Could you check a few things on this model? Use its own coordinates, in mm. Face numbers are marked on the shaded views. A direction names the side the tool comes from. Give positions to 0.01 mm unless a question says otherwise; leave off trailing zeros. Loops run counter-clockwise (first coordinate to the right, second up) from the corner with the lowest first, then second, coordinate; pieces in that order, holes last.
1. Imagine slicing it at D-D (x = 5). List the corners of the cut face in (y, z) for me.
2. Imagine slicing it at C-C (z = -21). List the corners of the cut face in (x, y) for me.
3. Imagine slicing it at B-B (y = -13). List the corners of the cut face in (x, z) for me.
4. For the marked faces 1, 2, 3 and 4, which set-ups out of +Z, -Z, +X, -X, +Y, -Y let a thin tool reach every point of the face, with its end or its side?
5. Thinking about a two-plate mould opening in Z: for the marked faces 5, 6 and 7, which applies, +Z half, -Z half, draft (parallel to the pull), parting line (faces both ways), or undercut?
6. I need wall thicknesses on line 1 along Y through (x, z) = (13.2, -21); line 2 along Z through (x, y) = (2.25, -5); line 3 along Z through (x, y) = (12.75, 1). Which ranges of each line are inside material? Lowest first, please.
7. Imagine slicing it at A-A (z = -4). List the corners of the cut face in (x, y) for me.
8. For P1, Ø1.2, axis at x = 0, y = 0, coming from the -Z side; P2, Ø3, axis at x = 11.5, z = -7.5, coming from the -Y side; P3, Ø1, axis at x = 9, z = -10, coming from the -Y side; P4, Ø5, axis at y = -13, z = 2, coming from the -X side, each with a flat end and sliding along its axis, tell me the tip position at first contact or that it passes through.
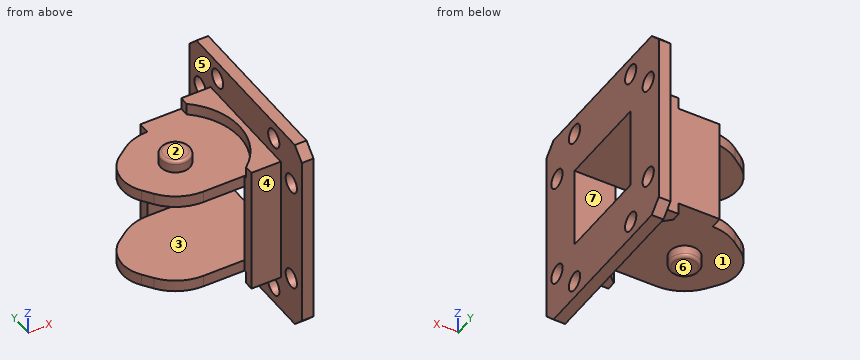
Autodesk Inventor part; units mm, degrees
ref_plane "Work Plane1" through (11, 0, 4) normal (1, 0, 0) x (0, 1, 0)
ref_plane "Work Plane2" through (0, 0, -7) normal (0, 0, -1) x (-1, 0, 0)
ref_plane "YZ Plane" through (0, 0, 0) normal (1, 0, 0) x (0, 1, 0)
sketch "Sketch1" plane through (0, 0, 0) normal (0, 0, 1) x (1, 0, 0)
  circle A0 centre (0, 0) radius 2.5
  circle A1 centre (20, 0) radius 2.5
  line L0 (7, 10) -> (20, 10)
  line L1 (7, -10) -> (20, -10)
  arc A2 (20, -10) -> (20, 10) centre (20, 0) ccw
  line L2 (7, 10) -> (7, 8)
  line L3 (7, -10) -> (7, -8)
  line L4 (7, 8) -> (0, 8)
  line L5 (7, -8) -> (0, -8)
  arc A3 (0, 8) -> (0, -8) centre (0, 0) ccw
  dimension "d0" = 5
  dimension "d1" = 20
  dimension "d2" = 10
  dimension "d3" = 2
  dimension "d4" = 13
extrude "Extrusion1" add sketch "Sketch1" along normal blind 4
sketch "Sketch2" plane through (0, 0, 4) normal (0, 0, 1) x (1, 0, 0)
  circle A0 centre (0, 0) radius 2.5
  line L0 (7, 8) -> (0, 8)
  arc A1 (0, 8) -> (0, -8) centre (0, 0) ccw
  line L1 (0, -8) -> (7, -8)
  line L2 (7, -10) -> (20, -10)
  line L3 (7, 8) -> (7, -8)
  line L4 (7, -8) -> (0, -8)
  line L5 (7, 8) -> (0, 8)
  arc A2 (0, 8) -> (0, -8) centre (0, 0) ccw
extrude "Extrusion2" cut sketch "Sketch2" against normal blind 2
sketch "Sketch3" plane through (0, 0, 0) normal (0, 0, -1) x (-1, 0, 0)
  circle A0 centre (-20, 0) radius 2.5
  circle A1 centre (0, 0) radius 2.5
  line L0 (-7, 10) -> (-20, 10)
  arc A2 (-20, 10) -> (-20, -10) centre (-20, 0) ccw
  line L1 (-20, -10) -> (-7, -10)
  line L2 (-7, 8) -> (-7, 10)
  line L3 (-19, 10) -> (-19, 8)
  line L4 (-19, 8) -> (-11, 8)
  line L5 (-11, 8) -> (-11, -8)
  line L6 (-11, -8) -> (-19, -8)
  line L7 (-19, -8) -> (-19, -10)
  point P0 (-7, -8)
  dimension "d9" = 1
  dimension "d10" = 11
extrude "Extrusion3" cut sketch "Sketch3" against normal blind 2 contours L3 L4 L5 L6 L7 L1 A2 L0
sketch "Sketch4" plane through (0, 0, 4) normal (0, 0, 1) x (1, 0, 0)
  line L0 (7, 10) -> (7, -10)
  circle A0 centre (0, 0) radius 2.5
  arc A1 (7, -8.485281) -> (7, 8.485281) centre (0, 0) ccw
  dimension "d15" = 11
extrude "Extrusion4" cut sketch "Sketch4" against normal blind 2 contours A1 L0
sketch "Sketch5" plane through (0, 0, 0) normal (0, 0, -1) x (-1, 0, 0)
  line L0 (0, 8) -> (-7, 8)
  line L1 (-7, 10) -> (0, 10)
  line L2 (0, 10) -> (0, 8)
  line L3 (0, 8) -> (-7, 8)
  line L4 (-7, 8) -> (-7, 10)
  arc A0 (0, -8) -> (0, 8) centre (0, 0) ccw
extrude "Extrusion5" add sketch "Sketch5" against normal blind 2
sketch "Sketch6" plane through (0, 0, 0) normal (0, 0, -1) x (-1, 0, 0)
  line L0 (0, 10) -> (-19, 10)
  line L1 (-19, 8) -> (-20, 8)
  line L2 (-20, 8) -> (-20, 10)
  line L3 (-20, 10) -> (-19, 10)
  line L4 (-19, 10) -> (-19, 8)
  circle A0 centre (-20, 0) radius 2.5
extrude "Extrusion6" add sketch "Sketch6" against normal blind 2 contours L1 L2 L3 L4
sketch "Sketch7" plane through (0, 0, 0) normal (0, 0, -1) x (-1, 0, 0)
  line L0 (-19, -8) -> (-19, -10)
  line L1 (-11, -8) -> (-19, -8)
  line L2 (-17.400642, -8) -> (-19, -9.162001)
  line L3 (-17.400642, -8) -> (-26.805206, 4.944272) construction
  line L4 (-26.805206, 4.944272) -> (-28.404564, 3.782271) construction
  line L5 (-28.404564, 3.782271) -> (-19, -9.162001) construction
  circle A0 centre (-20, 0) radius 2.5
  line L6 (-17.400642, -8) -> (-19, -8)
  line L7 (-19, -8) -> (-19, -9.162001)
  dimension "d21" = 16
  dimension "d22" = 8
  dimension "d23" = 36
extrude "Extrusion7" cut sketch "Sketch7" against normal blind 2 contours L1 L2 L0
sketch "Sketch9" plane through (0, 0, 2) normal (0, 0, 1) x (1, 0, 0)
  circle A0 centre (0, 0) radius 2.5
  arc A1 (11, 0) -> (7, 8.485281) centre (0, 0) ccw
  circle A2 centre (0, 0) radius 2.5
extrude "Extrusion8" add sketch "Sketch9" along normal mid plane 4
fillet "Fillet1" radius 0.5 1 edges at (-2.5, 0, 4)
sketch "Sketch10" plane through (0, 0, 0) normal (0, 0, -1) x (-1, 0, 0)
  arc A0 (0, -8) -> (0, 8) centre (0, 0) ccw
  line L0 (0, 10) -> (-20, 10)
  line L1 (4.702282, 6.472136) -> (11.174418, 1.769854)
  line L2 (11.174418, 1.769854) -> (6.472136, -4.702282)
  dimension "d30" = 144
extrude "Extrusion9" add sketch "Sketch10" against normal blind 2
fillet "Fillet2" radius 6 1 edges at (-11.1744, 1.7699, 1)
ref_plane "Work Plane1" through (11, 0, 4) normal (1, 0, 0) x (0, 1, 0)
split "Split1" plane through (11, 0, 4) removes the side toward (1, 0, 0)
sketch "Sketch11" plane through (11, -10, 0) normal (1, 0, 0) x (0, 0, -1)
  line L0 (0, 20) -> (0, 0)
  line L1 (-4, 20) -> (0, 20)
  line L2 (-4, 10) -> (-4, 20)
  line L3 (-4, 0) -> (-4, 10)
  line L4 (0, 0) -> (-4, 0)
  point P0 (0, 10)
extrude "Extrusion10" add sketch "Sketch11" along normal blind 1
ref_plane "Work Plane2" through (0, 0, -7) normal (0, 0, -1) x (-1, 0, 0)
mirror "Mirror1" about plane through (0, 0, -7) normal (0, 0, -1)
sketch "Sketch12" plane through (0, 0, 0) normal (0, 0, -1) x (-1, 0, 0)
  line L0 (-12, -10) -> (-7, -10)
  line L1 (-7, -10) -> (-7, -8)
  arc A0 (4.702282, 6.472136) -> (0, 8) centre (0, 0) ccw
  line L2 (0, 8) -> (0, 10)
  line L3 (0, 10) -> (-12, 10)
  line L4 (-12, -10) -> (-12, 10)
  line L5 (0, 8) -> (-12, 8)
  line L6 (-7, -8) -> (-12, -8)
extrude "Extrusion11" add sketch "Sketch12" along normal blind 14
sketch "Sketch17" plane through (12, -10, 0) normal (1, 0, 0) x (0, 0, -1)
  line L0 (0, 2) -> (0, 18)
  line L1 (0, 18) -> (14, 18)
  line L2 (14, 2) -> (14, 18)
  line L3 (0, 2) -> (14, 2)
  line L4 (18, 20) -> (18, 0)
  line L5 (-4, 20) -> (18, 20)
  line L6 (-4, 20) -> (-4, 0)
  line L7 (-8, 26) -> (22, 26)
  line L8 (24, 24) -> (24, -4)
  line L9 (22, -6) -> (-8, -6)
  line L10 (-10, -4) -> (-10, 24)
  line L11 (-7, 23) -> (21, 23) construction
  line L12 (21, 23) -> (21, -3) construction
  line L13 (21, -3) -> (-7, -3) construction
  line L14 (-7, -3) -> (-7, 23) construction
  circle A0 centre (-2, -3) radius 1.6
  circle A1 centre (16, -3) radius 1.6
  circle A2 centre (21, 2) radius 1.6
  circle A3 centre (21, 18) radius 1.6
  circle A4 centre (16, 23) radius 1.6
  circle A5 centre (-2, 23) radius 1.6
  circle A6 centre (-7, 18) radius 1.6
  circle A7 centre (-7, 2) radius 1.6
  line L15 (-10, 24) -> (-8, 26)
  line L16 (-10, -4) -> (-8, -6)
  line L17 (22, -6) -> (24, -4)
  line L18 (24, 24) -> (22, 26)
  point P0 (0, 10)
  point P1 (-10, 26)
  point P2 (24, -6)
  point P3 (24, 26)
  point P4 (-10, -6)
  point P5 (-7, 10)
  point P6 (-4, 10)
  point P7 (7, 23)
  point P8 (7, 20)
  point P9 (24, 10)
  point P10 (21, 10)
  point P11 (7, -6)
  point P12 (7, -3)
  dimension "d73" = 3.2
  dimension "d74" = 5
  dimension "d75" = 5
  dimension "d76" = 5
  dimension "d77" = 5
  dimension "d78" = 5
  dimension "d79" = 5
  dimension "d80" = 5
  dimension "d81" = 5
  dimension "d82" = 3
  dimension "d83" = 3
  dimension "d84" = 2
  dimension "d85" = 2
  dimension "d86" = 2
  dimension "d87" = 2
  dimension "d88" = 2
  dimension "d89" = 2
  dimension "d90" = 2
  dimension "d91" = 2
  dimension "d92" = 3
  dimension "d93" = 3
extrude "Extrusion16" add sketch "Sketch17" along normal blind 2
equation "\"d75\" = d74"
equation "\"d76\" = d75"
equation "\"d77\" = d76"
equation "\"d78\" = d76"
equation "\"d79\" = d75"
equation "\"d80\" = d75"
equation "\"d81\" = d75"
properties part number "z_axis_cable_mount_b" material "ABS Plastic"
Derived:
1. outline: (-8, -16) - (10, -16) - (10, 2) - (-8, 2) - (-8, 0) - (8, 0) - (8, -14) - (-8, -14) - close
2. outline: (12, -16) - (14, -16) - (14, -9.6) - (12, -9.6) - close; (12, -6.4) - (14, -6.4) - (14, 6.4) - (12, 6.4) - close; (12, 9.6) - (14, 9.6) - (14, 16) - (12, 16) - close
3. outline: (12, -24) - (14, -24) - (14, -17.6) - (12, -17.6) - close; (12, -14.4) - (14, -14.4) - (14, 0.4) - (12, 0.4) - close; (12, 3.6) - (14, 3.6) - (14, 10) - (12, 10) - close
4. face 1: -Z
4. face 2: +Z, -X, +Y, -Y
4. face 3: +X, -X
4. face 4: +Z, -Z, -X, -Y
5. face 5: draft
5. face 6: -Z half
5. face 7: undercut
6. line 1: y = -16 to -9.6, -6.4 to 6.4, 9.6 to 16
6. line 2: z = -16 to -14, 0 to 2
6. line 3: z = -24 to -14, 0 to 10
7. outline: (0, 8) - (14, 8) - (14, 16) - (12, 16) - (12, 10) - (0, 10) - close; (7, -10) - (12, -10) - (12, -16) - (14, -16) - (14, -8) - (7, -8) - close
8. P1: stops at z = -18
8. P2: stops at y = -16
8. P3: stops at y = -10
8. P4: stops at x = 12
